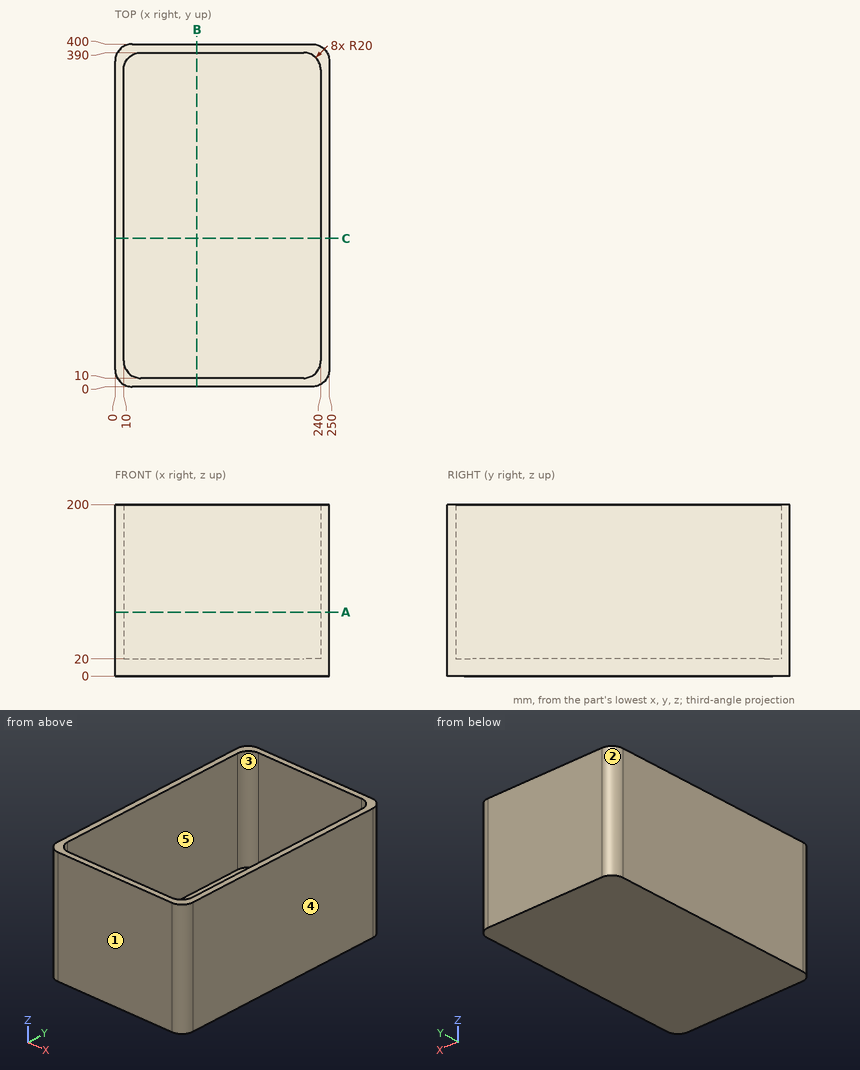
Could you check a few things on this drawing? It's one solid part, dimensions in mm from its lowest x, y, z. A direction names the side the tool comes from. Coordinates: 2 decimals unless noted, no trailing zeros. Write each loop counter-clockwise with the first axis right and the second up, starting at its lowest first coordinate (ties: lowest second). Pieces come first, ordered by that corner, then holes. Notation, with made-up numbers: (-5.5, 74) - (21.5, 74) arc R32 ccw to (21.5, 113) - close; hole circle Ø6 at (23.25, 65.25). An arc over 180 degrees is marked (long way). Use one line per item in the form item = value.
1) On a 3-axis mill with a long thin cutter (end or side, diameter ignored), from which of +Z, -Z, +X, -X, +Y, -Y can I reach the whole of each face in a straight line? I mean the marked faces 4 and 5. Say none if no direction works.
Solved:
face_4 = +Z, -Z, +X, +Y, -Y
face_5 = +Z
2) Suppose I cut it at C-C, the plane y = 173. Write out the boundary of the cut face in (x, z), plus the area to 3 significant figures.
Solved:
outline = (0, 0) - (250, 0) - (250, 200) - (240, 200) - (240, 20) - (10, 20) - (10, 200) - (0, 200) - close
area = 8,600 mm2
3) I need wall thicknesses on line 1 (Y direction, x = 63, z = 160); line 2 (X direction, y = 263, z = 182.5); line 3 (Z direction, x = 104, y = 220). Which ranges of each line are inside material? Lowest first, please.
Solved:
line_1 = 0 to 10, 390 to 400
line_2 = 0 to 10, 240 to 250
line_3 = 0 to 20
4) Thinking about a two-plate mould opening in X: for the marked faces 1, 2 and 3, which applies, released by +X, released by -X, zero draft, split by the parting line, or undercut?
Solved:
face_1 = zero draft
face_2 = released by -X
face_3 = undercut
5) Suppose I cut it at B-B, the plane x = 95.5. Write out the boundary of the cut face in (y, z).
Solved:
outline = (0, 0) - (400, 0) - (400, 200) - (390, 200) - (390, 20) - (10, 20) - (10, 200) - (0, 200) - close
6) Suppose I cut it at A-A, the plane z = 74.5. Write out the boundary of the cut face in (x, y), plus the area to 3 significant figures.
Solved:
outline = (0, 20) arc R20 ccw to (20, 0) - (230, 0) arc R20 ccw to (250, 20) - (250, 380) arc R20 ccw to (230, 400) - (20, 400) arc R20 ccw to (0, 380) - close; hole (10, 30) arc R20 ccw to (30, 10) - (220, 10) arc R20 ccw to (240, 30) - (240, 370) arc R20 ccw to (220, 390) - (30, 390) arc R20 ccw to (10, 370) - close
area = 12,600 mm2
7) I'm going to push a flat-ended pin straight in: P1, Ø12, axis at x = 112, y = 214.5, coming from the +Z side. Where does the tip first touch, or does it pass through?
Solved:
P1 = 20
